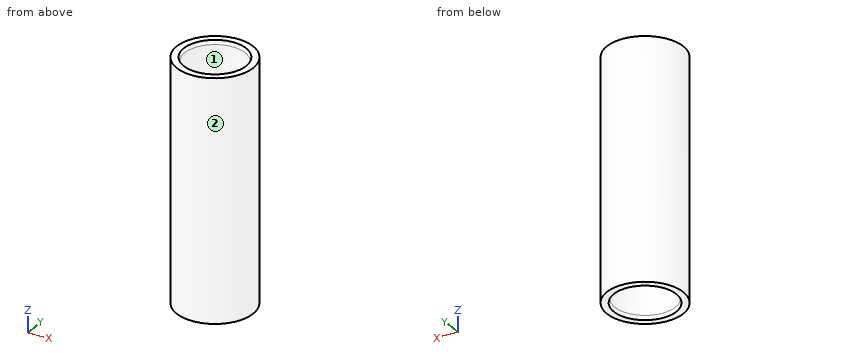
from build123d import *

# Parameters (mm, degrees)
SKETCH1_R           = 38
SKETCH1_R_2         = 30
BOSS_EXTRUDE1_DEPTH = 238
CHAMFER1_SIZE       = 4
CHAMFER1_SIZE2      = 1.07179677
CHAMFER2_SIZE       = 4
CHAMFER2_SIZE2      = 1.07179677


with BuildPart() as part:
    # Sketch1 → Boss-Extrude1 (new body)
    with BuildSketch(Plane.XY):
        Circle(SKETCH1_R)
        Circle(SKETCH1_R_2, mode=Mode.SUBTRACT)
    extrude(amount=BOSS_EXTRUDE1_DEPTH)

    # Chamfer1
    chamfer1_edges = [part.edges().sort_by_distance(p)[0] for p in [
        (-30, 0, 0),
    ]]
    chamfer1_side = [part.faces().sort_by_distance(p)[0] for p in [
        (-30, 0, 119),
    ]]
    chamfer(chamfer1_edges, length=CHAMFER1_SIZE, length2=CHAMFER1_SIZE2, reference=chamfer1_side[0])

    # Chamfer2
    chamfer2_edges = [part.edges().sort_by_distance(p)[0] for p in [
        (-30, 0, 238),
    ]]
    chamfer2_side = [part.faces().sort_by_distance(p)[0] for p in [
        (-30, 0, 121),
    ]]
    chamfer(chamfer2_edges, length=CHAMFER2_SIZE, length2=CHAMFER2_SIZE2, reference=chamfer2_side[0])


solid = part.part
For this review, take the finished solid that the model builds, in its own axes (mm). Face numbers are marked on the shaded views. Give positions to 0.01 mm unless a question says otherwise; leave off trailing zeros. Loops run counter-clockwise (first coordinate to the right, second up) from the corner with the lowest first, then second, coordinate; pieces in that order, holes last.
Item 1: Draft analysis for pull direction Y (two halves, no side actions). For the marked faces 1 and 2, state which applies: +Y half, -Y half, draft (parallel to the pull), parting line (faces both ways), or undercut.
Item 2: For line 1 along Y through (x, z) = (0, 104); line 2 along X through (y, z) = (-10, 108); line 3 along X through (y, z) = (-8, 141.5), list the stretches that pass through material, from the lowest coordinate up.
Item 3: Take a section at C-C, the plane y = 33.5. State the section outline as (x, z) points.
Item 4: Take a section at A-A, the plane x = 0. State the section outline as (y, z) points, and give its area (3 significant figures).
Item 5: Insertion check: pin 1 (4 mm diameter, centred on y = 16.5, z = 167, fed in from -X); pin 2 (1 mm diameter, centred on x = -13, z = 74.5, fed in from +Y); pin 3 (3 mm diameter, centred on x = -29.5, z = 194.5, fed in from +Y). Each pin has a flat end and moves straight along its axis. Give the tip position at first contact, or say it passes through.
Calculated:
1. face 1: undercut
1. face 2: parting line
2. line 1: y = -38 to -30, 30 to 38
2. line 2: x = -36.66 to -28.28, 28.28 to 36.66
2. line 3: x = -37.15 to -28.91, 28.91 to 37.15
3. outline: (-17.94, 0) - (17.94, 0) - (17.94, 238) - (-17.94, 238) - close
4. outline: (-38, 0) - (-31.07, 0) - (-30, 4) - (-30, 234) - (-31.07, 238) - (-38, 238) - close; (30, 4) - (31.07, 0) - (38, 0) - (38, 238) - (31.07, 238) - (30, 234) - close
4. area: 3,800 mm2
5. pin 1: stops at x = -35.12
5. pin 2: stops at y = 35.89
5. pin 3: stops at y = 25.69
